```python
from build123d import *

# Parameters (mm, degrees)
F0_W         = 50
F0_H         = 15
F2_DEPTH     = 2.4
F3_W         = 2.4
F3_H         = 15
F4_DEPTH     = 17.4
F6_T1_DEPTH  = 52.4
F5_R         = 1
F7_DEPTH     = 26.201
F8_T1_DEPTH  = 31.1484692284
F8_T3_DEPTH  = 31.1484692284
F8_T8_DEPTH  = 38.4969384567
F8_T13_DEPTH = 38.4969384567
F8_T18_DEPTH = 38.4969384567
F8_T23_DEPTH = 38.4969384567


# Not quite as in the source:
# - a fillet or chamfer that OpenCascade refuses, or shapes differently, is made with other operations: its cross-section is extruded or revolved along the edge and cut away or added


with BuildPart() as f2:
    # F0 (on Top) → F2 (new body)
    with BuildSketch(Plane.XY):
        Rectangle(F0_W, F0_H)
    extrude(amount=F2_DEPTH)

    # F3 (on face) → F4 (join)
    with BuildSketch(Plane.XY.offset(2.4)):
        Rectangle(F3_W, F3_H)
    extrude(amount=F4_DEPTH)

    # F6: fillet of radius 10 on 2 edges, made by hand

    # F6_s2 → F6_t1 (cut)
    with BuildSketch(Plane.YZ.offset(-26.2)):
        with BuildLine():
            ThreePointArc((-7.5, 9.8), (-4.5710678119, 16.8710678119), (2.5, 19.8))
            Line((2.5, 19.8), (-7.5, 19.8))
            Line((-7.5, 19.8), (-7.5, 9.8))
        make_face()
        with BuildLine():
            ThreePointArc((7.5, 9.8), (4.5710678119, 16.8710678119), (-2.5, 19.8))
            Line((-2.5, 19.8), (7.5, 19.8))
            Line((7.5, 19.8), (7.5, 9.8))
        make_face()
    extrude(amount=F6_T1_DEPTH, mode=Mode.SUBTRACT)

    # F5 (on face) → F7 (cut, through all)
    with BuildSketch(Plane.YZ.offset(1.2)):
        with Locations((0, 15.8)):
            Circle(F5_R)
    extrude(amount=-F7_DEPTH, mode=Mode.SUBTRACT)

    # F8: fillet of radius 3 on 4 edges, made by hand

    # F8_s2 → F8_t1 (cut)
    with BuildSketch(Plane.YZ.offset(-32.3484692284)):
        with BuildLine():
            ThreePointArc((-4.5606123087, 2.4), (-6.4579789048, 1.7237900077), (-7.5, 0))
            Line((-7.5, 0), (-7.5, 2.4))
            Line((-7.5, 2.4), (-4.5606123087, 2.4))
        make_face()
        with BuildLine():
            ThreePointArc((7.5, 0), (6.4579789048, 1.7237900077), (4.5606123087, 2.4))
            Line((4.5606123087, 2.4), (7.5, 2.4))
            Line((7.5, 2.4), (7.5, 0))
        make_face()
    extrude(amount=F8_T1_DEPTH, mode=Mode.SUBTRACT)

    # F8_s4 → F8_t3 (cut)
    with BuildSketch(Plane.YZ.offset(1.2)):
        with BuildLine():
            ThreePointArc((-4.5606123087, 2.4), (-6.4579789048, 1.7237900077), (-7.5, 0))
            Line((-7.5, 0), (-7.5, 2.4))
            Line((-7.5, 2.4), (-4.5606123087, 2.4))
        make_face()
        with BuildLine():
            ThreePointArc((7.5, 0), (6.4579789048, 1.7237900077), (4.5606123087, 2.4))
            Line((4.5606123087, 2.4), (7.5, 2.4))
            Line((7.5, 2.4), (7.5, 0))
        make_face()
    extrude(amount=F8_T3_DEPTH, mode=Mode.SUBTRACT)


with BuildPart() as f8_tool6:
    # F8_s7 → F8_t8 (new body)
    with BuildSketch(Plane.YZ.offset(-32.3484692284)):
        with BuildLine():
            ThreePointArc((-4.5606123087, 2.4), (-6.4579789048, 1.7237900077), (-7.5, 0))
            Line((-7.5, 0), (-7.5, 2.4))
            Line((-7.5, 2.4), (-4.5606123087, 2.4))
        make_face()
    extrude(amount=F8_T8_DEPTH)

    split(bisect_by=Plane.YZ.offset(1.2), keep=Keep.TOP)


with BuildPart() as f2_1:
    add(f2.part)

    # F8_t5: cut F8_tool6
    add(f8_tool6.part, mode=Mode.SUBTRACT)


with BuildPart() as f8_tool11:
    # F8_s12 → F8_t13 (new body)
    with BuildSketch(Plane.YZ.offset(-6.1484692284)):
        with BuildLine():
            ThreePointArc((-4.5606123087, 2.4), (-6.4579789048, 1.7237900077), (-7.5, 0))
            Line((-7.5, 0), (-7.5, 2.4))
            Line((-7.5, 2.4), (-4.5606123087, 2.4))
        make_face()
    extrude(amount=F8_T13_DEPTH)

    split(bisect_by=Plane.YZ.offset(-1.2), keep=Keep.BOTTOM)


with BuildPart() as f2_2:
    add(f2_1.part)

    # F8_t10: cut F8_tool11
    add(f8_tool11.part, mode=Mode.SUBTRACT)


with BuildPart() as f8_tool16:
    # F8_s17 → F8_t18 (new body)
    with BuildSketch(Plane.YZ.offset(32.3484692284)):
        with BuildLine():
            ThreePointArc((7.5, 0), (6.4579789048, 1.7237900077), (4.5606123087, 2.4))
            Line((4.5606123087, 2.4), (7.5, 2.4))
            Line((7.5, 2.4), (7.5, 0))
        make_face()
    extrude(amount=-F8_T18_DEPTH)

    split(bisect_by=Plane.YZ.offset(-1.2), keep=Keep.BOTTOM)


with BuildPart() as f2_3:
    add(f2_2.part)

    # F8_t15: cut F8_tool16
    add(f8_tool16.part, mode=Mode.SUBTRACT)


with BuildPart() as f8_tool21:
    # F8_s22 → F8_t23 (new body)
    with BuildSketch(Plane.YZ.offset(6.1484692284)):
        with BuildLine():
            ThreePointArc((7.5, 0), (6.4579789048, 1.7237900077), (4.5606123087, 2.4))
            Line((4.5606123087, 2.4), (7.5, 2.4))
            Line((7.5, 2.4), (7.5, 0))
        make_face()
    extrude(amount=-F8_T23_DEPTH)

    split(bisect_by=Plane.YZ.offset(1.2), keep=Keep.TOP)


with BuildPart() as f2_4:
    add(f2_3.part)

    # F8_t20: cut F8_tool21
    add(f8_tool21.part, mode=Mode.SUBTRACT)


solid = f2_4.part
```
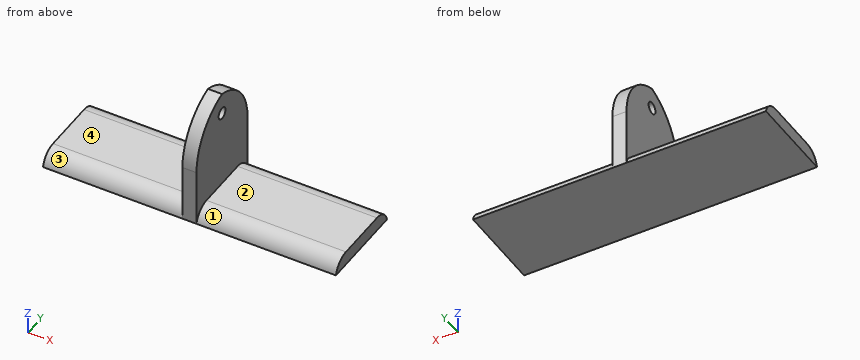
Could you check a few things on this model? Use its own coordinates, in mm. Face numbers are marked on the shaded views. A direction names the side the tool comes from. Give positions to 0.01 mm unless a question says otherwise; leave off trailing zeros. Loops run counter-clockwise (first coordinate to the right, second up) from the corner with the lowest first, then second, coordinate; pieces in that order, holes last. Notation, with made-up numbers: (0.5, 4) - (41.5, 4) arc R23 cw to (41.5, 21) - close; hole circle Ø11 at (24.25, -23). An arc over 180 degrees is marked (long way). Answer in a Markdown table with one row per item. Add a question column.
Q1. If we section it at A-A (z = 15.8): List the corners of the cut face in (x, y) for me.
Q2. For pin 1 (1.5 mm diameter, centred on y = 4.5, z = 11, fed in from +X); pin 2 (10 mm diameter, centred on x = 2.5, z = 17.5, fed in from -Y); pin 3 (7.5 mm diameter, centred on x = 15.5, y = 1, fed in from +Z), each with a flat end and sliding along its axis, tell me the tip position at first contact or that it passes through.
Q3. If we section it at C-C (y = -6): List the corners of the cut face in (x, z) for me.
Q4. If we section it at D-D (z = 5.5): List the corners of the cut face in (x, y) for me.
Q5. Please list where these lines run through material, in increasing order: L1, parallel to Z at x = -0.4, y = 0; L2, parallel to X at y = 5.75, z = 2.25; L3, parallel to Z at x = 14, y = 0.5. Write a range as from..to.
Q6. Which directions (+Z, -Z, +X, -X, +Y, -Y) give clear straight access to the entire face, cutting with the end or side of a thin tool? Please do the marked faces 1, 2, 3 and 4.
Q7. If we section it at B-B (y = -0.5): List the corners of the cut face in (x, z) for me, plus the area to 3 significant figures.
The answers:
| question | item | result |
|---|---|---|
| 1 | outline | (-1.2, -5.5) - (1.2, -5.5) - (1.2, -1) - (-1.2, -1) - close; (-1.2, 1) - (1.2, 1) - (1.2, 5.5) - (-1.2, 5.5) - close |
| 2 | pin 1 | stops at x = 1.2 |
| 2 | pin 2 | stops at y = -7.08 |
| 2 | pin 3 | stops at z = 2.4 |
| 3 | outline | (-25, 0) - (25, 0) - (25, 2.03) - (1.2, 2.03) - (1.2, 15.07) - (-1.2, 15.07) - (-1.2, 2.03) - (-25, 2.03) - close |
| 4 | outline | (-1.2, -7.5) - (1.2, -7.5) - (1.2, 7.5) - (-1.2, 7.5) - close |
| 5 | L1 | z = 0..14.8, 16.8..19.48 |
| 5 | L2 | x = -1.2..1.2 |
| 5 | L3 | z = 0..2.4 |
| 6 | face 1 | +Z, +X, -Y |
| 6 | face 2 | +Z, +X, +Y, -Y |
| 6 | face 3 | +Z, -X, -Y |
| 6 | face 4 | +Z, -X, +Y, -Y |
| 7 | outline | (-25, 0) - (25, 0) - (25, 2.4) - (1.2, 2.4) - (1.2, 14.93) - (-1.2, 14.93) - (-1.2, 2.4) - (-25, 2.4) - close; (-1.2, 16.67) - (1.2, 16.67) - (1.2, 19.34) - (-1.2, 19.34) - close |
| 7 | area | 156 mm^2 |
